Input: part model. Units: mm. Frame: model coordinates. Give positions to 0.01 mm unless a question says otherwise; leave off trailing zeros. Order: outer loops, then holes, each group sorted by start corner. A loop starts at its lowest first (then second) coordinate and runs counter-clockwise, first axis right, second up. Notation, with made-up numbers: (-1, 23.5) - (15, 23.5) arc R35 ccw to (15, 61.5) - close; hole circle Ø11 at (6.5, -29). An arc over 180 degrees is marked (long way). Answer in a Markdown table with one row per item. Add a question column.
1. Contact query for flat-ended pins moving along their axis: pin 1 (2 mm diameter, centred on x = 13.5, z = 97.5, fed in from -Y); pin 2 (1.5 mm diameter, centred on x = 13.5, y = 20, fed in from +Z). Output: stop coordinate, or through.
2. Ray query, line 1 (Z direction, x = 9, y = 0.5); line 2 (Y direction, x = 14, z = 31.5); line 3 (Y direction, x = 13.25, z = -6.5). Return the intervals inside material, ascending. Write a range as [from, to].
3. Section query A-A on z = 104. Return loops of the section in (x, y).
4. Section query B-B on z = 79.5. Return loops of the section in (x, y).
```python
from build123d import *

# Parameters (mm, degrees)
BASPROSKE_W         = 15
BASPROSKE_H         = 22
TOOTHCUT_DEPTH      = 35.539832078
TEETHCUTS_COUNT     = 20
TEETHCUTS_ANGLE     = 342
BORSKE_R            = 0.5
BORE_DEPTH          = 50.0000508
SKETCH1_R           = 11.1
CUT_EXTRUDE1_DEPTH  = 16
CUT_EXTRUDE2_DEPTH  = 8
SKETCH3_R           = 11.1
BOSS_EXTRUDE2_DEPTH = 7
SKETCH5_W           = 56.998857039
SKETCH5_H           = 22.722114901
CUT_EXTRUDE3_DEPTH  = 7
SKETCH6_R           = 17.499
BOSS_EXTRUDE3_DEPTH = 7
SKETCH7_R           = 1.7
CUT_EXTRUDE4_DEPTH  = 7
BOSS_EXTRUDE5_DEPTH = 7


with BuildPart() as part:
    # BasProSke → Base-Revolve (revolve)
    with BuildSketch(Plane(origin=(0, 0, 0), x_dir=(1, 0, 0), z_dir=(0, 1, 0)), mode=Mode.PRIVATE) as base_revolve_sk:
        with Locations((7.5, 11)):
            Rectangle(BASPROSKE_W, BASPROSKE_H)
    revolve(base_revolve_sk.sketch.rotate(Axis((-10, 0, 0), (1, 0, 0)), 180), axis=Axis((-10, 0, 0), (1, 0, 0)))

    # TooCutSke → ToothCut (cut, through all)
    with BuildSketch(Plane(origin=(0, 0, 0), x_dir=(0, 0, -1), z_dir=(1, 0, 0))):
        with BuildLine():
            ThreePointArc((0.986171591, 17.471189616), (0, 17.499), (-0.986171591, 17.471189616))
            ThreePointArc((-0.986171591, 17.471189616), (-1.626916196, 19.798789858), (-2.932850173, 21.829260982))
            ThreePointArc((-2.932850173, 21.829260982), (0, 22.0254), (2.932850173, 21.829260982))
            ThreePointArc((2.932850173, 21.829260982), (1.626916196, 19.798789858), (0.986171591, 17.471189616))
        make_face()
    toothcut = extrude(amount=TOOTHCUT_DEPTH, mode=Mode.SUBTRACT)

    # TeethCuts: ToothCut ×20 about axis
    teethcuts_axis = Axis((-10, 0, 0), (1, 0, 0))
    for i in range(1, TEETHCUTS_COUNT):
        add(toothcut.rotate(teethcuts_axis, i * TEETHCUTS_ANGLE / (TEETHCUTS_COUNT - 1)), mode=Mode.SUBTRACT)

    # BorSke → Bore (cut, symmetric)
    with BuildSketch(Plane(origin=(0, 0, 0), x_dir=(0, 0, -1), z_dir=(1, 0, 0))):
        with Locations(Location((0, 0, 0), (0, 0, 180))):
            Circle(BORSKE_R)
    extrude(amount=BORE_DEPTH, both=True, mode=Mode.SUBTRACT)

    # Sketch1 → Cut-Extrude1 (cut)
    with BuildSketch(Plane.ZY):
        Circle(SKETCH1_R)
    extrude(amount=-CUT_EXTRUDE1_DEPTH, mode=Mode.SUBTRACT)

    # Sketch2 → Cut-Extrude2 (cut)
    with BuildSketch(Plane.ZY):
        with BuildLine():
            ThreePointArc((17.471189616, 0.986171591), (19.784848102, 1.620704589), (21.806333941, 2.912696354))
            ThreePointArc((21.806333941, 2.912696354), (21.729143493, 3.441558231), (21.639128664, 3.968388926))
            ThreePointArc((21.639128664, 3.968388926), (19.317333972, 4.572472634), (16.920832513, 4.460989585))
            ThreePointArc((16.920832513, 4.460989585), (16.642537979, 5.407488385), (16.31134495, 6.336799421))
            ThreePointArc((16.31134495, 6.336799421), (18.31568345, 7.655235955), (19.838983319, 9.50866662))
            ThreePointArc((19.838983319, 9.50866662), (19.602143532, 9.987790994), (19.353734704, 10.461020648))
            ThreePointArc((19.353734704, 10.461020648), (16.958904602, 10.318064378), (14.714146429, 9.471478019))
            ThreePointArc((14.714146429, 9.471478019), (14.156988385, 10.28565413), (13.554832194, 11.067137173))
            ThreePointArc((13.554832194, 11.067137173), (15.05365209, 12.940419489), (15.929654782, 15.173862347))
            ThreePointArc((15.929654782, 15.173862347), (15.556349186, 15.556349186), (15.173862347, 15.929654782))
            ThreePointArc((15.173862347, 15.929654782), (12.940419489, 15.05365209), (11.067137173, 13.554832194))
            ThreePointArc((11.067137173, 13.554832194), (10.28565413, 14.156988385), (9.471478019, 14.714146429))
            ThreePointArc((9.471478019, 14.714146429), (10.318064378, 16.958904602), (10.461020648, 19.353734704))
            ThreePointArc((10.461020648, 19.353734704), (9.987790994, 19.602143532), (9.50866662, 19.838983319))
            ThreePointArc((9.50866662, 19.838983319), (7.655235955, 18.31568345), (6.336799421, 16.31134495))
            ThreePointArc((6.336799421, 16.31134495), (5.407488385, 16.642537979), (4.460989585, 16.920832513))
            ThreePointArc((4.460989585, 16.920832513), (4.572472634, 19.317333972), (3.968388926, 21.639128664))
            ThreePointArc((3.968388926, 21.639128664), (3.441558231, 21.729143493), (2.912696354, 21.806333941))
            ThreePointArc((2.912696354, 21.806333941), (1.620704589, 19.784848102), (0.986171591, 17.471189616))
            ThreePointArc((0.986171591, 17.471189616), (0, 17.499), (-0.986171591, 17.471189616))
            ThreePointArc((-0.986171591, 17.471189616), (-1.620704589, 19.784848102), (-2.912696354, 21.806333941))
            ThreePointArc((-2.912696354, 21.806333941), (-3.441558231, 21.729143493), (-3.968388926, 21.639128664))
            ThreePointArc((-3.968388926, 21.639128664), (-4.572472634, 19.317333972), (-4.460989585, 16.920832513))
            ThreePointArc((-4.460989585, 16.920832513), (-5.407488385, 16.642537979), (-6.336799421, 16.31134495))
            ThreePointArc((-6.336799421, 16.31134495), (-7.655235955, 18.31568345), (-9.50866662, 19.838983319))
            ThreePointArc((-9.50866662, 19.838983319), (-9.987790994, 19.602143532), (-10.461020648, 19.353734704))
            ThreePointArc((-10.461020648, 19.353734704), (-10.318064378, 16.958904602), (-9.471478019, 14.714146429))
            ThreePointArc((-9.471478019, 14.714146429), (-10.28565413, 14.156988385), (-11.067137173, 13.554832194))
            ThreePointArc((-11.067137173, 13.554832194), (-12.940419489, 15.05365209), (-15.173862347, 15.929654782))
            ThreePointArc((-15.173862347, 15.929654782), (-15.556349186, 15.556349186), (-15.929654782, 15.173862347))
            ThreePointArc((-15.929654782, 15.173862347), (-15.05365209, 12.940419489), (-13.554832194, 11.067137173))
            ThreePointArc((-13.554832194, 11.067137173), (-14.156988385, 10.28565413), (-14.714146429, 9.471478019))
            ThreePointArc((-14.714146429, 9.471478019), (-16.958904602, 10.318064378), (-19.353734704, 10.461020648))
            ThreePointArc((-19.353734704, 10.461020648), (-19.602143532, 9.987790994), (-19.838983319, 9.50866662))
            ThreePointArc((-19.838983319, 9.50866662), (-18.31568345, 7.655235955), (-16.31134495, 6.336799421))
            ThreePointArc((-16.31134495, 6.336799421), (-16.642537979, 5.407488385), (-16.920832513, 4.460989585))
            ThreePointArc((-16.920832513, 4.460989585), (-19.317333972, 4.572472634), (-21.639128664, 3.968388926))
            ThreePointArc((-21.639128664, 3.968388926), (-21.729143493, 3.441558231), (-21.806333941, 2.912696354))
            ThreePointArc((-21.806333941, 2.912696354), (-19.784848102, 1.620704589), (-17.471189616, 0.986171591))
            ThreePointArc((-17.471189616, 0.986171591), (-17.499, 0), (-17.471189616, -0.986171591))
            ThreePointArc((-17.471189616, -0.986171591), (-19.784848102, -1.620704589), (-21.806333941, -2.912696354))
            ThreePointArc((-21.806333941, -2.912696354), (-21.729143493, -3.441558231), (-21.639128664, -3.968388926))
            ThreePointArc((-21.639128664, -3.968388926), (-19.317333972, -4.572472634), (-16.920832513, -4.460989585))
            ThreePointArc((-16.920832513, -4.460989585), (-16.642537979, -5.407488385), (-16.31134495, -6.336799421))
            ThreePointArc((-16.31134495, -6.336799421), (-18.31568345, -7.655235955), (-19.838983319, -9.50866662))
            ThreePointArc((-19.838983319, -9.50866662), (-19.602143532, -9.987790994), (-19.353734704, -10.461020648))
            ThreePointArc((-19.353734704, -10.461020648), (-16.958904602, -10.318064378), (-14.714146429, -9.471478019))
            ThreePointArc((-14.714146429, -9.471478019), (-14.156988385, -10.28565413), (-13.554832194, -11.067137173))
            ThreePointArc((-13.554832194, -11.067137173), (-15.05365209, -12.940419489), (-15.929654782, -15.173862347))
            ThreePointArc((-15.929654782, -15.173862347), (-15.556349186, -15.556349186), (-15.173862347, -15.929654782))
            ThreePointArc((-15.173862347, -15.929654782), (-12.940419489, -15.05365209), (-11.067137173, -13.554832194))
            ThreePointArc((-11.067137173, -13.554832194), (-10.28565413, -14.156988385), (-9.471478019, -14.714146429))
            ThreePointArc((-9.471478019, -14.714146429), (-10.318064378, -16.958904602), (-10.461020648, -19.353734704))
            ThreePointArc((-10.461020648, -19.353734704), (-9.987790994, -19.602143532), (-9.50866662, -19.838983319))
            ThreePointArc((-9.50866662, -19.838983319), (-7.655235955, -18.31568345), (-6.336799421, -16.31134495))
            ThreePointArc((-6.336799421, -16.31134495), (-5.407488385, -16.642537979), (-4.460989585, -16.920832513))
            ThreePointArc((-4.460989585, -16.920832513), (-4.572472634, -19.317333972), (-3.968388926, -21.639128664))
            ThreePointArc((-3.968388926, -21.639128664), (-3.441558231, -21.729143493), (-2.912696354, -21.806333941))
            ThreePointArc((-2.912696354, -21.806333941), (-1.620704589, -19.784848102), (-0.986171591, -17.471189616))
            ThreePointArc((-0.986171591, -17.471189616), (0, -17.499), (0.986171591, -17.471189616))
            ThreePointArc((0.986171591, -17.471189616), (1.620704589, -19.784848102), (2.912696354, -21.806333941))
            ThreePointArc((2.912696354, -21.806333941), (3.441558231, -21.729143493), (3.968388926, -21.639128664))
            ThreePointArc((3.968388926, -21.639128664), (4.572472634, -19.317333972), (4.460989585, -16.920832513))
            ThreePointArc((4.460989585, -16.920832513), (5.407488385, -16.642537979), (6.336799421, -16.31134495))
            ThreePointArc((6.336799421, -16.31134495), (7.655235955, -18.31568345), (9.50866662, -19.838983319))
            ThreePointArc((9.50866662, -19.838983319), (9.987790994, -19.602143532), (10.461020648, -19.353734704))
            ThreePointArc((10.461020648, -19.353734704), (10.318064378, -16.958904602), (9.471478019, -14.714146429))
            ThreePointArc((9.471478019, -14.714146429), (10.28565413, -14.156988385), (11.067137173, -13.554832194))
            ThreePointArc((11.067137173, -13.554832194), (12.940419489, -15.05365209), (15.173862347, -15.929654782))
            ThreePointArc((15.173862347, -15.929654782), (15.556349186, -15.556349186), (15.929654782, -15.173862347))
            ThreePointArc((15.929654782, -15.173862347), (15.05365209, -12.940419489), (13.554832194, -11.067137173))
            ThreePointArc((13.554832194, -11.067137173), (14.156988385, -10.28565413), (14.714146429, -9.471478019))
            ThreePointArc((14.714146429, -9.471478019), (16.958904602, -10.318064378), (19.353734704, -10.461020648))
            ThreePointArc((19.353734704, -10.461020648), (19.602143532, -9.987790994), (19.838983319, -9.50866662))
            ThreePointArc((19.838983319, -9.50866662), (18.31568345, -7.655235955), (16.31134495, -6.336799421))
            ThreePointArc((16.31134495, -6.336799421), (16.642537979, -5.407488385), (16.920832513, -4.460989585))
            ThreePointArc((16.920832513, -4.460989585), (19.317333972, -4.572472634), (21.639128664, -3.968388926))
            ThreePointArc((21.639128664, -3.968388926), (21.729143493, -3.441558231), (21.806333941, -2.912696354))
            ThreePointArc((21.806333941, -2.912696354), (19.784848102, -1.620704589), (17.471189616, -0.986171591))
            ThreePointArc((17.471189616, -0.986171591), (17.499, 0), (17.471189616, 0.986171591))
        make_face()
    extrude(amount=-CUT_EXTRUDE2_DEPTH, mode=Mode.SUBTRACT)

    # Sketch3 → Boss-Extrude2 (add)
    with BuildSketch(Plane.ZY.offset(-8)):
        Circle(SKETCH3_R)
    extrude(amount=-BOSS_EXTRUDE2_DEPTH)

    # Sketch5 → Cut-Extrude3 (cut)
    with BuildSketch(Plane.ZY.offset(-8)):
        with Locations((-1.101858783, 11.361057451)):
            Rectangle(SKETCH5_W, SKETCH5_H)
    extrude(amount=-CUT_EXTRUDE3_DEPTH, mode=Mode.SUBTRACT)

    # Sketch6 → Boss-Extrude3 (add)
    with BuildSketch(Plane.ZY.offset(-8)):
        Circle(SKETCH6_R)
    extrude(amount=-BOSS_EXTRUDE3_DEPTH)

    # Sketch7 → Cut-Extrude4 (cut)
    with BuildSketch(Plane.ZY.offset(-8)):
        Circle(SKETCH7_R)
    extrude(amount=-CUT_EXTRUDE4_DEPTH, mode=Mode.SUBTRACT)

    # Sketch8 → Boss-Extrude5 (add)
    with BuildSketch(Plane.ZY.offset(-8)):
        with BuildLine():
            Line((64.951905284, 54.999), (0, 17.499))
            ThreePointArc((0, 17.499), (12.267429085, 12.478989729), (17.496442259, 0.299180999))
            Line((17.496442259, 0.299180999), (71.26903982, 31.344804676))
            Line((71.26903982, 31.344804676), (86.167351448, 27.352814106))
            Line((86.167351448, 27.352814106), (112.148113562, 42.352814106))
            Line((112.148113562, 42.352814106), (64.951905284, 54.999))
        make_face()
    extrude(amount=-BOSS_EXTRUDE5_DEPTH)


solid = part.part
```
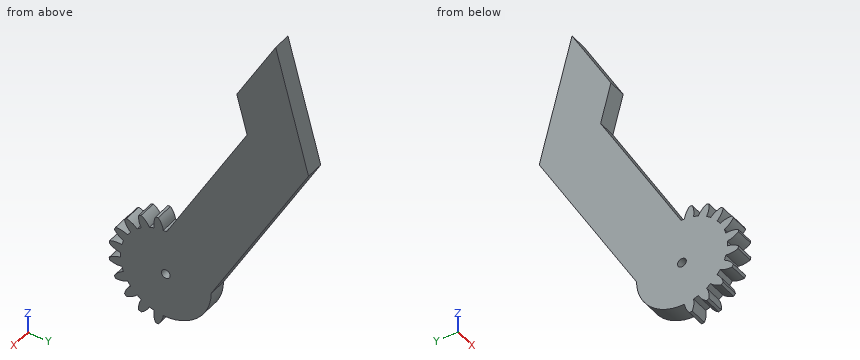
Answer:
| question | item | result |
|---|---|---|
| 1 | pin 1 | stops at y = 33.32 |
| 1 | pin 2 | stops at z = 52.92 |
| 2 | line 1 | z = [-17.49, -1.62], [1.62, 17.84] |
| 2 | line 2 | y = [8.38, 35.69] |
| 2 | line 3 | y = [-16.65, 16.25] |
| 3 | outline | (8, 37.65) - (15, 37.65) - (15, 44.54) - (8, 44.54) - close |
| 4 | outline | (8, 29.14) - (15, 29.14) - (15, 51.1) - (8, 51.1) - close |
